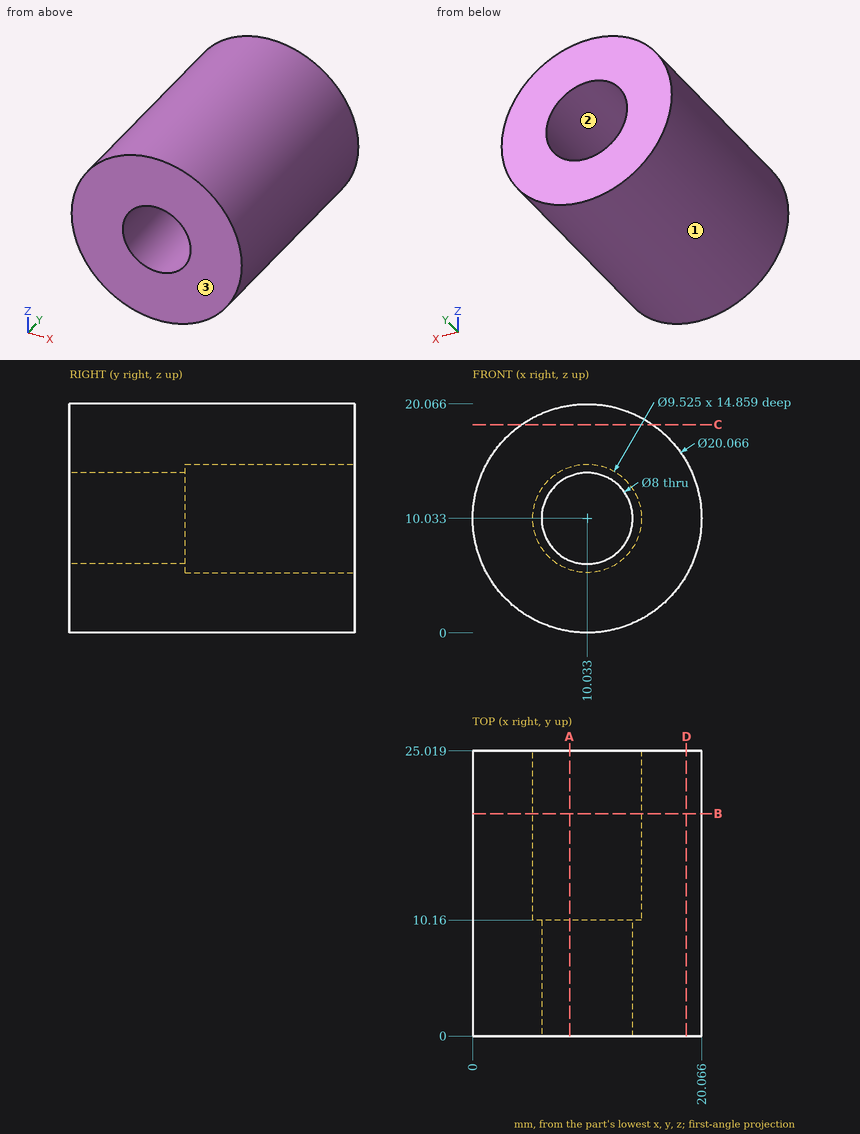
Can you work these out from the drawing? Everything is in mm from the part's minimum corner. Round coordinates to 2 decimals unless told otherwise and drop trailing zeros. Write each loop counter-clockwise with the first axis right and the second up, starting at its lowest first coordinate (ties: lowest second). Pieces come first, ordered by that corner, then holes.
1. Suppose I cut it at D-D (x = 18.75). List the corners of the cut face in (y, z) for me.
2. Suppose I cut it at C-C (z = 18.25). List the corners of the cut face in (x, y) for me.
3. Will these pins go through, and if not, where does the flat tip stop? pin 1 Ø1.5 at (y, z) = (17.5, 16.5) entering from +X; pin 2 Ø10 at (x, y) = (4, 3.5) entering from +Z; pin 3 Ø5 at (x, y) = (14.5, 17.5) entering from -Z.
4. If we mould it in two halves opening along X, with no side actions, what happens to the marked faces 1, 2 and 3? For each: released by +X, released by -X, zero draft, split by the parting line, or undercut.
5. I need wall thicknesses on L1, parallel to Z at x = 9.25, y = 23; L2, parallel to X at y = 19, z = 11; L3, parallel to X at y = 4, z = 9.5. Which ranges of each line are inside material? Lowest first, please.
6. Suppose I cut it at A-A (x = 8.5). List the corners of the cut face in (y, z) for me.
7. Suppose I cut it at B-B (y = 19.5). List the corners of the cut face in (x, z) for me (1 decimal).
Answer sheet:
1. outline: (0, 5.07) - (25.02, 5.07) - (25.02, 15) - (0, 15) - close
2. outline: (4.28, 0) - (15.79, 0) - (15.79, 25.02) - (4.28, 25.02) - close
3. pin 1: stops at x = 18.28
3. pin 2: stops at z = 20.01
3. pin 3: stops at z = 0.19
4. face 1: split by the parting line
4. face 2: undercut
4. face 3: zero draft
5. L1: z = 0.03 to 5.34, 14.73 to 20.04
5. L2: x = 0.05 to 5.37, 14.7 to 20.02
5. L3: x = 0.01 to 6.07, 14 to 20.05
6. outline: (0, 0.12) - (25.02, 0.12) - (25.02, 5.52) - (10.16, 5.52) - (10.16, 6.34) - (0, 6.34) - close; (0, 13.73) - (10.16, 13.73) - (10.16, 14.54) - (25.02, 14.54) - (25.02, 19.95) - (0, 19.95) - close
7. outline: circle Ø20.1 at (10, 10); hole circle Ø9.5 at (10, 10)
